Work out the finished part from the listing and answer in its coordinate system (mm). A direction names the side the tool comes from. Coordinates: 2 decimals unless noted, no trailing zeros. Write each loop counter-clockwise with the first axis right and the second up, starting at its lowest first coordinate (ties: lowest second). Pieces come first, ordered by that corner, then holes. Notation, with made-up numbers: (-40, 57) - (-32, 57) arc R9 ccw to (-32, 63) - close; hole circle Ø3 at (-34, 13). An arc over 180 degrees is marked (long way). Answer as a JSON object with one key per item and string values. Group by question number.
from build123d import *
from build123d.topology import SkipClean

# Parameters (mm, degrees)
EXTRUDE_1_DEPTH     = 200
SKETCH_4_R          = 5
CUT_EXTRUDE_3_DEPTH = 5
SKETCH_5_R          = 5
CUT_EXTRUDE_4_DEPTH = 5
SKETCH_6_R          = 71
CUT_EXTRUDE_5_DEPTH = 10
SKETCH_7_R          = 71
CUT_EXTRUDE_6_DEPTH = 10


with BuildPart() as part:
    # 草图1 → 凸台-拉伸1 (new body)
    with BuildSketch(Plane(origin=(0, 0, 0), x_dir=(0, 0, -1), z_dir=(1, 0, 0))):
        Polygon((141.421356237, 141.421356237), (0, 0), (200, 0), (200, 4), (9.656854249, 4), (144.249783362, 138.592929113), align=None)
    extrude(amount=EXTRUDE_1_DEPTH)

    # 草图4 → 切除-拉伸3 (cut)
    with SkipClean():  # the faces are left unmerged after this step: merging them gives an invalid solid
        with BuildSketch(Plane(origin=(0, 0, 0), x_dir=(1, 0, 0), z_dir=(0, 0.7071067811865512, 0.7071067811865438))):
            with Locations(Location((12.5, 150, 0), (0, 0, 270))):
                Circle(SKETCH_4_R)
            with Locations(Location((12.5, 50, 0), (0, 0, 270))):
                Circle(SKETCH_4_R)
            with Locations(Location((50, 187.5, 0), (0, 0, 270))):
                Circle(SKETCH_4_R)
            with Locations(Location((150, 187.5, 0), (0, 0, 270))):
                Circle(SKETCH_4_R)
            with Locations(Location((187.5, 50, 0), (0, 0, 270))):
                Circle(SKETCH_4_R)
            with Locations(Location((187.5, 150, 0), (0, 0, 270))):
                Circle(SKETCH_4_R)
            with Locations(Location((150, 12.5, 0), (0, 0, 325.345312559))):
                Circle(SKETCH_4_R)
            with Locations(Location((50, 12.5, 0), (0, 0, 325.345312559))):
                Circle(SKETCH_4_R)
        extrude(amount=-CUT_EXTRUDE_3_DEPTH, mode=Mode.SUBTRACT)

    # 草图5 → 切除-拉伸4 (cut)
    with BuildSketch(Plane.XZ):
        with Locations(Location((12.5, -50, 0), (0, 0, 270))):
            Circle(SKETCH_5_R)
        with Locations(Location((12.5, -150, 0), (0, 0, 270))):
            Circle(SKETCH_5_R)
        with Locations(Location((50, -187.5, 0), (0, 0, 270))):
            Circle(SKETCH_5_R)
        with Locations(Location((150, -187.5, 0), (0, 0, 270))):
            Circle(SKETCH_5_R)
        with Locations(Location((150, -12.5, 0), (0, 0, 34.654687441))):
            Circle(SKETCH_5_R)
        with Locations(Location((50, -12.5, 0), (0, 0, 34.654687441))):
            Circle(SKETCH_5_R)
        with Locations(Location((187.5, -150, 0), (0, 0, 270))):
            Circle(SKETCH_5_R)
        with Locations(Location((187.5, -50, 0), (0, 0, 270))):
            Circle(SKETCH_5_R)
    extrude(amount=-CUT_EXTRUDE_4_DEPTH, mode=Mode.SUBTRACT)

    # 草图6 → 切除-拉伸5 (cut)
    with BuildSketch(Plane(origin=(0, 0, 0), x_dir=(1, 0, 0), z_dir=(0, 0.7071067811865512, 0.7071067811865439))):
        with Locations(Location((100, 100, 0), (0, 0, 270))):
            Circle(SKETCH_6_R)
    extrude(amount=-CUT_EXTRUDE_5_DEPTH, mode=Mode.SUBTRACT)

    # 草图7 → 切除-拉伸6 (cut)
    with BuildSketch(Plane.XZ):
        with Locations(Location((100, -100, 0), (0, 0, 270))):
            Circle(SKETCH_7_R)
    extrude(amount=-CUT_EXTRUDE_6_DEPTH, mode=Mode.SUBTRACT)


solid = part.part
Q1. Section B-B on x = 150 is taken. Determine the outline of the cut face in (y, z), plus the area to 3 significant figures.
Q2. Section C-C on x = 100 is taken. Determine the outline of the cut face in (y, z), plus the area to 3 significant figures.
Q3. Section D-D on x = 187.5 is taken. Determine the outline of the cut face in (y, z), plus the area to 3 significant figures.
Q4. Section A-A on z = -187.5 is taken. Determine the outline of the cut face in (x, y).
Q5. Flat-ended cylindrical pins translate along their axes: pin 1 Ø13 at (x, z) = (50, -12.5) entering from +Y; pin 2 Ø10 at (x, y) = (169, 55.5) entering from -Z; pin 3 Ø8 at (x, z) = (50, -187.5) entering from -Y; pin 4 Ø10 at (x, z) = (77.5, -133.5) entering from +Y. Find the tip coordinate at first contact, or state that the pin passes through.
Q6. Consider L1, parallel to X at y = 2.6, z = -187.5; L2, parallel to X at y = 0.8, z = -100; L3, parallel to X at y = 1, z = -150. Determine where each line is inside the solid, lowest interval first. Write a range as from..to.
Q7. A tool of negligible diameter and unlimited length cuts with its end or side. For faces 1 (the face through (170.4, 2, -90.8)), 2 (the face through (170.396, 75.852, -78.641)), from which of +Z, -Z, +X, -X, +Y, -Y can it reach the whole face along a straight path? Write none if from no direction.
Q8. For a pull along X with two mould halves and no side action, classify faces 3 (the face through (145.119, 131.955, -134.743)), 4 (the face through (200, 3, -92)), 5 (the face through (76, 119, -119)) as +X half, -X half, draft (parallel to the pull), parting line (faces both ways), or undercut.
Numbers:
{
 "1": {"outline": "(0, -200) - (4, -200) - (4, -192.5) - (0, -192.5) - close; (0, -182.5) - (4, -182.5) - (4, -150.41) - (0, -150.41) - close; (0, -49.59) - (4, -49.59) - (4, -17.5) - (0, -17.5) - close; (0, -7.5) - (3.11, -7.5) - (5.3, -5.3) - (0, 0) - close; (9.55, -15.2) - (32.24, -37.9) - (35.07, -35.07) - (12.37, -12.37) - close; (103.53, -109.18) - (126.22, -131.88) - (129.05, -129.05) - (106.35, -106.35) - close; (133.29, -138.95) - (138.59, -144.25) - (141.42, -141.42) - (136.12, -136.12) - close", "area": "597 mm²"},
 "2": {"outline": "(0, -200) - (4, -200) - (4, -171) - (0, -171) - close; (0, -29) - (4, -29) - (4, -9.66) - (17.68, -23.33) - (20.51, -20.51) - (0, 0) - close; (118.09, -123.74) - (138.59, -144.25) - (141.42, -141.42) - (120.92, -120.92) - close", "area": "425 mm²"},
 "3": {"outline": "(0, -200) - (4, -200) - (4, -155) - (0, -155) - close; (0, -145) - (4, -145) - (4, -55) - (0, -55) - close; (0, -45) - (4, -45) - (4, -9.66) - (28.99, -34.65) - (31.82, -31.82) - (0, 0) - close; (36.06, -41.72) - (99.7, -105.36) - (102.53, -102.53) - (38.89, -38.89) - close; (106.77, -112.43) - (138.59, -144.25) - (141.42, -141.42) - (109.6, -109.6) - close", "area": "1,400 mm²"},
 "4": {"outline": "(0, 0) - (45, 0) - (45, 4) - (0, 4) - close; (55, 0) - (145, 0) - (145, 4) - (55, 4) - close; (155, 0) - (200, 0) - (200, 4) - (155, 4) - close"},
 "5": {"pin 1": "stops at y = 19", "pin 2": "stops at z = -66.01", "pin 3": "passes through", "pin 4": "stops at y = 138.5"},
 "6": {"L1": "x = 0..45, 55..145, 155..200", "L2": "x = 0..29, 171..200", "L3": "x = 0..7.5, 17.5..49.59, 150.41..182.5, 192.5..200"},
 "7": {"face 1": "-Y", "face 2": "none"},
 "8": {"face 3": "undercut", "face 4": "+X half", "face 5": "draft"}
}
